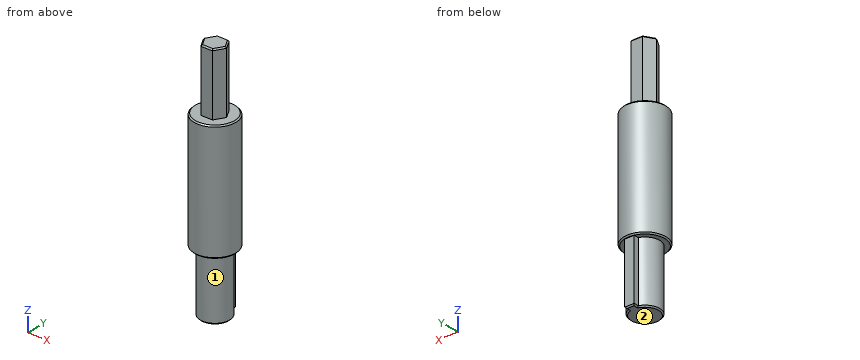
```python
from build123d import *

# Parameters (mm, degrees)
SKETCH2_R           = 6
BOSS_EXTRUDE1_DEPTH = 25.4
BOSS_EXTRUDE2_START = 25
BOSS_EXTRUDE2_DEPTH = 25
SKETCH4_R           = 8.5
BOSS_EXTRUDE3_DEPTH = 48
BOSS_EXTRUDE4_DEPTH = 25.4
CHAMFER1_SIZE       = 0.5


with BuildPart() as part:
    # Sketch2 → Boss-Extrude1 (new body)
    with BuildSketch(Plane.XY):
        Circle(SKETCH2_R)
    extrude(amount=BOSS_EXTRUDE1_DEPTH)

    # Sketch3 → Boss-Extrude2 (add)
    with BuildSketch(Plane(origin=(0, 0, 0), x_dir=(-1, 0, 0), z_dir=(0, 0, -1)).offset(BOSS_EXTRUDE2_START)):
        with BuildLine():
            Line((-1.95, 5.674284096), (-1.95, 7.674284096))
            Line((-1.95, 7.674284096), (1.95, 7.674284096))
            Line((1.95, 7.674284096), (1.95, 5.674284096))
            ThreePointArc((1.95, 5.674284096), (0, -6), (-1.95, 5.674284096))
        make_face()
    extrude(amount=-BOSS_EXTRUDE2_DEPTH)

    # Sketch4 → Boss-Extrude3 (add)
    with BuildSketch(Plane.XY):
        Circle(SKETCH4_R)
    extrude(amount=BOSS_EXTRUDE3_DEPTH)

    # Sketch5 → Boss-Extrude4 (add)
    with BuildSketch(Plane.XY.offset(48)):
        Polygon((4.766026472, 0), (2.383013236, 4.1275), (-2.383013236, 4.1275), (-4.766026472, 0), (-2.383013236, -4.1275), (2.383013236, -4.1275), align=None)
    extrude(amount=BOSS_EXTRUDE4_DEPTH)

    # Chamfer1
    chamfer1_edges = [part.edges().sort_by_distance(p)[0] for p in [
        (-8.5, 0, 0),
        (-8.5, 0, 48),
        (3.574519854, -2.06375, 73.4),
        (3.574519854, 2.06375, 73.4),
        (0, 4.1275, 73.4),
        (-3.574519854, 2.06375, 73.4),
        (-3.574519854, -2.06375, 73.4),
        (0, -4.1275, 73.4),
        (0, -6, -25),
        (-1.95, 6.674284096, -25),
        (0, 7.674284096, -25),
        (1.95, 6.674284096, -25),
    ]]
    chamfer(chamfer1_edges, length=CHAMFER1_SIZE)


solid = part.part
```
Geometry check sheet. Reference: the model listing, model coordinates, mm. Face numbers are marked on the shaded views. A direction names the side the tool comes from. Coordinates: 2 decimals unless noted, no trailing zeros. Loops run counter-clockwise (first coordinate to the right, second up) from the corner with the lowest first, then second, coordinate; pieces in that order, holes last. Notation, with made-up numbers: (22.5, -2) - (56.5, -2) arc R19 ccw to (56.5, 8) - close; hole circle Ø11 at (27, 42). An arc over 180 degrees is marked (long way). One line per item, written item: value. Start each with the question number.
(1) Tool access check on the marked faces 1 and 2. Record the directions out of +Z, -Z, +X, -X, +Y, -Y that give a thin tool (end or side, any length) a straight path to the whole face; none if there is none.
(2) Cross-section at C-C on z = 54. Enter the section's corners in (x, y), plus the area to 3 significant figures.
(3) Cross-section at B-B on z = 13.5. Enter the section's corners in (x, y).
(4) Depth check by flat-ended pin: P1, Ø1, axis at x = -3, z = 11, coming from the -Y side; P2, Ø3, axis at x = 1.5, z = 55.5, coming from the -Y side; P3, Ø4, axis at x = -6.5, z = -12, coming from the +Y side. Enter the tip coordinate at first touch or a pass-through.
(5) Material ranges on line 1 (X direction, y = 7.5, z = -8.5); line 2 (Y direction, x = 6, z = 12); line 3 (X direction, y = 1, z = 49), recorded low to high. Write a range as [from, to].
(6) Cross-section at A-A on x = 0. Enter the section's corners in (y, z).
Results below:
1. face 1: -Z
1. face 2: -Z, +X, -X, +Y, -Y
2. outline: (-4.77, 0) - (-2.38, -4.13) - (2.38, -4.13) - (4.77, 0) - (2.38, 4.13) - (-2.38, 4.13) - close
2. area: 59.0 mm2
3. outline: circle Ø17 at (0, 0)
4. P1: stops at y = -8.12
4. P2: stops at y = -4.13
4. P3: stops at y = 3.97
5. line 1: x = [-1.95, 1.95]
5. line 2: y = [-6.02, 6.02]
5. line 3: x = [-4.19, 4.19]
6. outline: (-8.5, 0.5) - (-8, 0) - (-6, 0) - (-6, -24.5) - (-5.5, -25) - (7.17, -25) - (7.67, -24.5) - (7.67, 0) - (8, 0) - (8.5, 0.5) - (8.5, 47.5) - (8, 48) - (4.13, 48) - (4.13, 72.9) - (3.63, 73.4) - (-3.63, 73.4) - (-4.13, 72.9) - (-4.13, 48) - (-8, 48) - (-8.5, 47.5) - close
